```python
from build123d import *

# Parameters (mm, degrees)
F1_DEPTH = 152.4
F2_W     = 317.5
F2_H     = 218.3699290887
F3_DEPTH = 152.4
F4_R     = 63.5
F5_DEPTH = 127
F6_R     = 63.5
F7_DEPTH = 127


with BuildPart() as f1:
    # F0 (on Top) → F1 (new body)
    with BuildSketch(Plane.XY):
        Polygon((0, 317.5), (0, 0), (1016, 0), (1016, 635), (0, 635), align=None)
        with BuildLine():
            ThreePointArc((266.7, 317.5), (190.5, 241.3), (114.3, 317.5))
            ThreePointArc((114.3, 317.5), (190.5, 393.7), (266.7, 317.5))
        make_face(mode=Mode.SUBTRACT)
        with BuildLine():
            ThreePointArc((711.2, 317.5), (635, 241.3), (558.8, 317.5))
            ThreePointArc((558.8, 317.5), (635, 393.7), (711.2, 317.5))
        make_face(mode=Mode.SUBTRACT)
    extrude(amount=F1_DEPTH)

    # F2 (on face) → F3 (join)
    with BuildSketch(Plane.YZ.offset(1016)):
        with BuildLine():
            Line((317.5, 370.7699290887), (635, 370.7699290887))
            Line((635, 370.7699290887), (508, 787.4))
            Line((508, 787.4), (406.4, 787.4))
            Line((406.4, 787.4), (406.4, 533.4))
            ThreePointArc((406.4, 533.4), (380.3617928475, 470.5382071525), (317.5, 444.5))
            Line((317.5, 444.5), (317.5, 370.7699290887))
        make_face()
        with Locations((476.25, 261.5849645443)):
            Rectangle(F2_W, F2_H)
        with Locations((158.75, 261.5849645443)):
            Rectangle(F2_W, F2_H)
        with BuildLine():
            Line((127, 787.4), (0, 370.7699290887))
            Line((0, 370.7699290887), (317.5, 370.7699290887))
            Line((317.5, 370.7699290887), (317.5, 444.5))
            ThreePointArc((317.5, 444.5), (254.6382071525, 470.5382071525), (228.6, 533.4))
            Line((228.6, 533.4), (228.6, 787.4))
            Line((228.6, 787.4), (127, 787.4))
        make_face()
    extrude(amount=-F3_DEPTH)

    # F4 (on face) → F5 (join)
    with BuildSketch(Plane.XZ):
        with BuildLine():
            Line((1016, 370.7699290887), (1016, 0))
            Line((1016, 0), (1193.8, 0))
            ThreePointArc((1193.8, 0), (1344.3065953325, 128.4516229901), (1241.1016888122, 297.273428328))
            Line((1241.1016888122, 297.273428328), (1016, 370.7699290887))
        make_face()
        with Locations((1193.8, 152.4)):
            Circle(F4_R, mode=Mode.SUBTRACT)
    extrude(amount=-F5_DEPTH)

    # F6 (on face) → F7 (join)
    with BuildSketch(Plane(origin=(0, 635, 0), x_dir=(-1, 0, 0), z_dir=(0, 1, 0))):
        with BuildLine():
            Line((-1016, 0), (-1016, 370.7699290887))
            Line((-1016, 370.7699290887), (-1241.1016888122, 297.273428328))
            ThreePointArc((-1241.1016888122, 297.273428328), (-1344.3065953325, 128.4516229901), (-1193.8, 0))
            Line((-1193.8, 0), (-1016, 0))
        make_face()
        with Locations((-1193.8, 152.4)):
            Circle(F6_R, mode=Mode.SUBTRACT)
    extrude(amount=-F7_DEPTH)


solid = f1.part
```
For this review, take the finished solid that the model builds, in its own axes (mm). A direction names the side the tool comes from. Round coordinates to 2 decimals unless told otherwise and drop trailing zeros. Write each loop counter-clockwise with the first axis right and the second up, starting at its lowest first coordinate (ties: lowest second). Pieces come first, ordered by that corner, then holes. Notation, with made-up numbers: (61.25, -32) -> (72.25, -32) arc R26 ccw to (72.25, 0) -> close; hole circle Ø1 at (55, 78.25). An arc over 180 degrees is marked (long way). Use one line per item in the form item = value.
Q1. Machinability: for faces 1 (the flat face through (1105, 127, 188)), 2 (the flat face through (863.6, 313, 404)), 3 (the flat face through (941, 179, 787.4)), 4 (the flat face through (941, 228.6, 659)), 5 (the flat face through (1016, 313, 399)), which of the approach directions +Z, -Z, +X, -X, +Y, -Y give a long, thin tool a straight path to every point of the face, cutting with its end or side? Answer none if there is none.
Resolved:
face_1 = +Z, -Z, +X
face_2 = +Z, -X, +Y, -Y
face_3 = +Z, +X, -X, +Y, -Y
face_4 = +Z, +X, -X
face_5 = +Z, +X
Q2. Clearance check with flat-ended pins moving along their axes: pin 1 Ø2 at (x, y) = (767, 313) entering from +Z; pin 2 Ø4 at (x, y) = (684.5, 391) entering from -Z; pin 3 Ø10 at (y, z) = (207, 185.5) entering from +X; pin 4 Ø12 at (y, z) = (225, 280) entering from -X. State where each tip first meets the part, or that it passes through.
Resolved:
pin_1 = 152.4
pin_2 = 0
pin_3 = 1016
pin_4 = 863.6
Q3. To check wall thickness, follow probe 1 along Y at (x, z) = (190.5, 56); probe 2 along Z at (x, y) = (521, 350.5); probe 3 along X at (y, z) = (360, 148.5). State the ranges of each line that lie inside material, in increasing order. Write a range as from..to.
Resolved:
probe_1 = 0..241.3, 393.7..635
probe_2 = 0..152.4
probe_3 = 0..127.25, 253.75..571.75, 698.25..1016
Q4. The part is to be moulded in two halves that separate along Y. For faces 6 (the flat face through (832, 635, 147)), 7 (the flat face through (605, 393, 0)), 8 (the cylindrical face through (155.338, 249.897, 75.133)), say which applies: released by +Y, released by -Y, zero draft, split by the parting line, or undercut.
Resolved:
face_6 = released by +Y
face_7 = zero draft
face_8 = undercut
Q5. Consider section B-B (z = 126.5). State the section outline as (x, y) points, then the cut area to 3 significant figures.
Resolved:
outline = (0, 0) -> (1135.82, 0) -> (1135.82, 127) -> (1016, 127) -> (1016, 508) -> (1135.82, 508) -> (1135.82, 635) -> (0, 635) -> close; (1251.78, 0) -> (1343.98, 0) -> (1343.98, 127) -> (1251.78, 127) -> close; (1251.78, 508) -> (1343.98, 508) -> (1343.98, 635) -> (1251.78, 635) -> close; hole circle Ø152.4 at (190.5, 317.5); hole circle Ø152.4 at (635, 317.5)
area = 663,000 mm²
Q6. Consider section D-D (y = 590.5). State the section outline as (x, z) points.
Resolved:
outline = (0, 0) -> (1193.8, 0) arc R152.4 ccw to (1241.1, 297.27) -> (1016, 370.77) -> (1016, 516.75) -> (863.6, 516.75) -> (863.6, 152.4) -> (0, 152.4) -> close; hole circle Ø127 at (1193.8, 152.4)
Q7. Consider section A-A (y = 255). State the section outline as (x, z) points.
Resolved:
outline = (0, 0) -> (146.91, 0) -> (146.91, 152.4) -> (0, 152.4) -> close; (234.09, 0) -> (591.41, 0) -> (591.41, 152.4) -> (234.09, 152.4) -> close; (678.59, 0) -> (1016, 0) -> (1016, 470.18) -> (863.6, 470.18) -> (863.6, 152.4) -> (678.59, 152.4) -> close
Q8. Consider section C-C (x = 1079). State the section outline as (y, z) points.
Resolved:
outline = (0, 0) -> (127, 0) -> (127, 350.2) -> (0, 350.2) -> close; (508, 0) -> (635, 0) -> (635, 350.2) -> (508, 350.2) -> close
